Model file for the job. Use its own axes, mm. Round coordinates to 2 decimals unless told otherwise and drop trailing zeros. Loops run counter-clockwise (first coordinate to the right, second up) from the corner with the lowest first, then second, coordinate; pieces in that order, holes last. Notation, with made-up numbers: M -21.5,-37 L -10.5,-37 A23 ccw -10.5,-14 Z; hole C 22,50 d4. An arc over 180 degrees is marked long. Use a Markdown table: item, result. Add a question column.
Q1. Cut at C-C (z = -22.5). Give the cut face in (x, y).
Q2. Cut at A-A (y = 7.5). State how many separate pieces and enclosed holes the cut face has, plus the area to 3 significant figures.
Q3. Cut at D-D (x = 57). Give the cut face in (y, z), plus the area to 3 significant figures.
Q4. Probe line 1 (X direction, y = 1, z = 0); line 2 (X direction, y = 2.75, z = -35); line 3 (X direction, y = 1.45, z = -32.5). List the from-to ranges inside material, lowest first. Write a range as from..to.
Q5. Pin check, flat tips, straight feed: pin 1 (3 mm diameter, centred on x = 30, z = -32.5, fed in from +Y); pin 2 (3 mm diameter, centred on x = -83, z = 33.5, fed in from -Y). Stop position of each tip, or through.
Q6. Cut at B-B (x = -68). Give the cut face in (y, z).
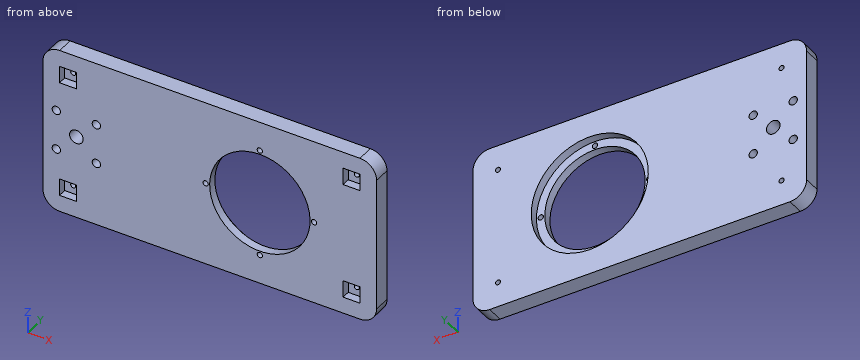
from build123d import *

# Parameters (mm, degrees)
SKETCH_1_W          = 200
SKETCH_1_H          = 100
EXTRUDE_1_DEPTH     = 10
SKETCH_2_R          = 2.5
SKETCH_2_R_2        = 30.1
SKETCH_2_R_3        = 4.1
CUT_EXTRUDE_1_DEPTH = 113.249721603
SKETCH_3_R          = 35.1
CUT_EXTRUDE_2_DEPTH = 5
FILLET_1_R          = 10
SKETCH_4_W          = 10.2
SKETCH_4_H          = 10.2
CUT_EXTRUDE_4_DEPTH = 5
SKETCH_5_R          = 1.6
CUT_EXTRUDE_5_DEPTH = 112.915146428
SKETCH_6_R          = 1.5
CUT_EXTRUDE_7_DEPTH = 113.249721603


with BuildPart() as part:
    # Sketch 1 → Extrude 1 (new body)
    with BuildSketch(Plane(origin=(0, 0, 0), x_dir=(1, 0, 0), z_dir=(0, 1, 0))):
        Rectangle(SKETCH_1_W, SKETCH_1_H)
    extrude(amount=EXTRUDE_1_DEPTH)

    # Sketch 2 → Cut-Extrude 1 (cut, through all)
    with BuildSketch(Plane(origin=(0, 10, 0), x_dir=(1, 0, 0), z_dir=(0, 1, 0))):
        with Locations(Location((-92, 12, 0), (0, 0, 270))):
            Circle(SKETCH_2_R)
        with Locations(Location((-68, 12, 0), (0, 0, 270))):
            Circle(SKETCH_2_R)
        with Locations(Location((-92, -12, 0), (0, 0, 270))):
            Circle(SKETCH_2_R)
        with Locations(Location((-68, -12, 0), (0, 0, 270))):
            Circle(SKETCH_2_R)
        with Locations(Location((30, 0, 0), (0, 0, 270))):
            Circle(SKETCH_2_R_2)
        with Locations(Location((-80, 0, 0), (0, 0, 270))):
            Circle(SKETCH_2_R_3)
    extrude(amount=-CUT_EXTRUDE_1_DEPTH, mode=Mode.SUBTRACT)

    # Sketch 3 → Cut-Extrude 2 (cut)
    with BuildSketch(Plane.XZ.offset(-10)):
        with Locations(Location((30, 0, 0), (0, 0, 270))):
            Circle(SKETCH_3_R)
    extrude(amount=CUT_EXTRUDE_2_DEPTH, mode=Mode.SUBTRACT)

    # Fillet 1
    fillet_1_edges = [part.edges().sort_by_distance(p)[0] for p in [
        (100, 5, 50),
        (-100, 5, 50),
        (-100, 5, -50),
        (100, 5, -50),
    ]]
    fillet(fillet_1_edges, radius=FILLET_1_R)

    # Sketch 4 → Cut-Extrude 4 (cut)
    with BuildSketch(Plane.XZ):
        with Locations((-85, 35)):
            Rectangle(SKETCH_4_W, SKETCH_4_H)
        with Locations((-85, -35)):
            Rectangle(SKETCH_4_W, SKETCH_4_H)
        with Locations((85, 35)):
            Rectangle(SKETCH_4_W, SKETCH_4_H)
        with Locations((85, -35)):
            Rectangle(SKETCH_4_W, SKETCH_4_H)
    extrude(amount=-CUT_EXTRUDE_4_DEPTH, mode=Mode.SUBTRACT)

    # Sketch 5 → Cut-Extrude 5 (cut, through all)
    with BuildSketch(Plane(origin=(0, 5, 0), x_dir=(1, 0, 0), z_dir=(0, 1, 0))):
        with Locations(Location((-2.5, 0, 0), (0, 0, 270))):
            Circle(SKETCH_5_R)
        with Locations(Location((62.5, 0, 0), (0, 0, 270))):
            Circle(SKETCH_5_R)
        with Locations(Location((30, 32.5, 0), (0, 0, 270))):
            Circle(SKETCH_5_R)
        with Locations(Location((30, -32.5, 0), (0, 0, 270))):
            Circle(SKETCH_5_R)
    extrude(amount=-CUT_EXTRUDE_5_DEPTH, mode=Mode.SUBTRACT)

    # Sketch 6 → Cut-Extrude 7 (cut, through all)
    with BuildSketch(Plane(origin=(0, 0, 0), x_dir=(1, 0, 0), z_dir=(0, 1, 0))):
        with Locations(Location((-85, -35, 0), (0, 0, 270))):
            Circle(SKETCH_6_R)
        with Locations(Location((-85, 35, 0), (0, 0, 270))):
            Circle(SKETCH_6_R)
        with Locations(Location((85, 35, 0), (0, 0, 270))):
            Circle(SKETCH_6_R)
        with Locations(Location((85, -35, 0), (0, 0, 270))):
            Circle(SKETCH_6_R)
    extrude(amount=CUT_EXTRUDE_7_DEPTH, mode=Mode.SUBTRACT)


solid = part.part
Checked values:
| question | item | result |
|---|---|---|
| 1 | outline | M -100,0 L 10.01,0 L 10.01,5 L 3.06,5 L 3.06,10 L -100,10 Z; M 49.99,0 L 100,0 L 100,10 L 56.94,10 L 56.94,5 L 49.99,5 Z |
| 2 | separate pieces | 1 |
| 2 | enclosed holes | 10 |
| 2 | area | 15,900 mm^2 |
| 3 | outline | M 0,-50 L 10,-50 L 10,-22.43 L 5,-22.43 L 5,-13.3 L 0,-13.3 Z; M 0,13.3 L 5,13.3 L 5,22.43 L 10,22.43 L 10,50 L 0,50 Z |
| 3 | area | 643 mm^2 |
| 4 | line 1 | x = -100..-84.1, -75.9..-4.1, -0.9..-0.1, 60.1..60.9, 64.1..100 |
| 4 | line 2 | x = -100..-90.1, -79.9..79.9, 90.1..100 |
| 4 | line 3 | x = -100..-90.1, -79.9..28.4, 31.6..79.9, 90.1..100 |
| 5 | pin 1 | passes through |
| 5 | pin 2 | stops at y = 5 |
| 6 | outline | M 0,-50 L 10,-50 L 10,-14.5 L 0,-14.5 Z; M 0,-9.5 L 10,-9.5 L 10,9.5 L 0,9.5 Z; M 0,14.5 L 10,14.5 L 10,50 L 0,50 Z |
